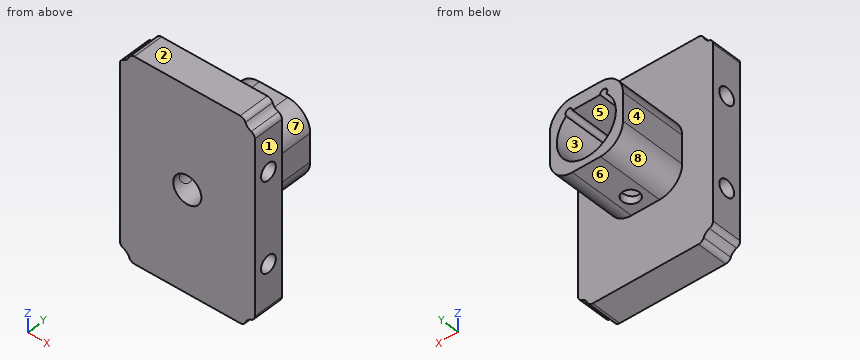
from build123d import *

# Parameters (mm, degrees)
EXTRUDE_1_DEPTH     = 12
EXTRUDE_3_DEPTH     = 5.5
SKETCH_6_R          = 1.5
CUT_EXTRUDE_2_DEPTH = 31
SKETCH_7_R          = 1.5
CUT_EXTRUDE_3_DEPTH = 31
SKETCH_8_R          = 2.5
CUT_EXTRUDE_5_DEPTH = 31
EXTRUDE_START       = -24
SKETCH_9_R          = 1.5
EXTRUDE_4_DEPTH     = 24
SKETCH_10_R         = 2.5
CUT_EXTRUDE_6_DEPTH = 24


with BuildPart() as part:
    # 草图1 → 凸台-拉伸1 (new body)
    with BuildSketch(Plane(origin=(0, 0, 0), x_dir=(1, 0, 0), z_dir=(0, 1, 0))):
        with BuildLine():
            ThreePointArc((6.5, -2.5), (5.328427125, -5.328427125), (2.5, -6.5))
            Line((2.5, -6.5), (-2.5, -6.5))
            ThreePointArc((-2.5, -6.5), (-5.328427125, -5.328427125), (-6.5, -2.5))
            Line((-6.5, -2.5), (-6.5, 2.5))
            ThreePointArc((-6.5, 2.5), (-5.328427125, 5.328427125), (-2.5, 6.5))
            Line((-2.5, 6.5), (2.5, 6.5))
            ThreePointArc((2.5, 6.5), (5.328427125, 5.328427125), (6.5, 2.5))
            Line((6.5, 2.5), (6.5, -2.5))
        make_face()
        with BuildLine():
            ThreePointArc((3.581278005, -3.838873253), (0, 5.25), (-3.581278005, -3.838873253))
            ThreePointArc((-3.581278005, -3.838873253), (-3.300605298, -4.858604348), (-2.435602742, -4.25))
            Line((-2.435602742, -4.25), (2.435602742, -4.25))
            ThreePointArc((2.435602742, -4.25), (3.300605298, -4.858604348), (3.581278005, -3.838873253))
        make_face(mode=Mode.SUBTRACT)
    extrude(amount=EXTRUDE_1_DEPTH)

    # 草图3 → 凸台-拉伸3 (add)
    with BuildSketch(Plane.XZ):
        with BuildLine():
            Line((12, 15.394651328), (12, -15.394651328))
            ThreePointArc((12, -15.394651328), (11.824116747, -15.961071302), (11.358336826, -16.328243701))
            ThreePointArc((11.358336826, -16.328243701), (10.733804764, -16.733804764), (10.328243701, -17.358336826))
            ThreePointArc((10.328243701, -17.358336826), (9.961071302, -17.824116747), (9.394651328, -18))
            Line((9.394651328, -18), (-9.394651328, -18))
            ThreePointArc((-9.394651328, -18), (-9.961071302, -17.824116747), (-10.328243701, -17.358336826))
            ThreePointArc((-10.328243701, -17.358336826), (-10.733804764, -16.733804764), (-11.358336826, -16.328243701))
            ThreePointArc((-11.358336826, -16.328243701), (-11.824116747, -15.961071302), (-12, -15.394651328))
            Line((-12, -15.394651328), (-12, 15.394651328))
            ThreePointArc((-12, 15.394651328), (-11.824116747, 15.961071302), (-11.358336826, 16.328243701))
            ThreePointArc((-11.358336826, 16.328243701), (-10.733804764, 16.733804764), (-10.328243701, 17.358336826))
            ThreePointArc((-10.328243701, 17.358336826), (-9.961071302, 17.824116747), (-9.394651328, 18))
            Line((-9.394651328, 18), (9.394651328, 18))
            ThreePointArc((9.394651328, 18), (9.961071302, 17.824116747), (10.328243701, 17.358336826))
            ThreePointArc((10.328243701, 17.358336826), (10.733804764, 16.733804764), (11.358336826, 16.328243701))
            ThreePointArc((11.358336826, 16.328243701), (11.824116747, 15.961071302), (12, 15.394651328))
        make_face()
    extrude(amount=EXTRUDE_3_DEPTH)

    # 草图6 → 切除-拉伸2 (cut)
    with BuildSketch(Plane.ZY.offset(12)):
        with Locations((0, -2.75)):
            Circle(SKETCH_6_R)
        with Locations((8, -2.75)):
            Circle(SKETCH_6_R)
        with Locations((-8, -2.75)):
            Circle(SKETCH_6_R)
    extrude(amount=-CUT_EXTRUDE_2_DEPTH, mode=Mode.SUBTRACT)

    # 草图7 → 切除-拉伸3 (cut)
    with BuildSketch(Plane.XY.offset(6.5)):
        with Locations((0, 3)):
            Circle(SKETCH_7_R)
    extrude(amount=-CUT_EXTRUDE_3_DEPTH, mode=Mode.SUBTRACT)

    # 草图8 → 切除-拉伸5 (cut)
    with BuildSketch(Plane.XZ.offset(5.5)):
        with Locations(Location((0, 0, 0), (0, 0, 270))):
            Circle(SKETCH_8_R)
    extrude(amount=-CUT_EXTRUDE_5_DEPTH, mode=Mode.SUBTRACT)

    # 草图9 → 凸台-拉伸4 (add)
    with BuildSketch(Plane(origin=(12, 0, 0), x_dir=(0, 0, -1), z_dir=(1, 0, 0)).offset(EXTRUDE_START)):
        with Locations(Location((0, -2.75, 0), (0, 0, 180))):
            Circle(SKETCH_9_R)
    extrude(amount=EXTRUDE_4_DEPTH)

    # 草图10 → 切除-拉伸6 (cut)
    with BuildSketch(Plane.XZ.offset(5.5)):
        with Locations(Location((0, 0, 0), (0, 0, 270))):
            Circle(SKETCH_10_R)
    extrude(amount=-CUT_EXTRUDE_6_DEPTH, mode=Mode.SUBTRACT)


solid = part.part
Design review of the part built by this model. Coordinates are the model's own, in mm. Face numbers are marked on the shaded views. A direction names the side the tool comes from. Give positions to 0.01 mm unless a question says otherwise; leave off trailing zeros. Order: outer loops, then holes, each group sorted by start corner. A loop starts at its lowest first (then second) coordinate and runs counter-clockwise, first axis right, second up. Notation, with made-up numbers: (-10, -19) - (10, -19) arc R18 ccw to (10, -8) - close; hole circle Ø5 at (-11, 27). An arc over 180 degrees is marked (long way). Use CSV: the item, a comma, the result in double quotes. Start each with the question number.
Q1. Take a section at C-C (y = -2.75). State the section outline as (x, z) points.
Q2. Take a section at D-D (z = 0). State the section outline as (x, y) points.
Q3. Draft analysis for pull direction X (two halves, no side actions). For the marked faces 1, 2 and 3, state which applies: pulls with the +X half, pulls with the -X half, needs draft (parallel to the pull), parting line crosses it, or undercut.
Q4. For line 1 (Y direction, x = 3.5, z = 8); line 2 (Z direction, x = 0, y = 6.25); line 3 (Z direction, x = -7, y = -3.75), list the stretches that pass through material, from the lowest coordinate up.
Q5. Machinability: for the marked faces 4, 5, 6, 7 and 8, which of the approach directions +Z, -Z, +X, -X, +Y, -Y give a long, thin tool a straight path to every point of the face, cutting with its end or side? Answer none if there is none.
Q6. Take a section at A-A (x = 0). State the section outline as (y, z) points.
Q7. Take a section at B-B (z = 8). State the section outline as (x, y) points, and give its area (3 significant figures).
Q8. For P1, Ø3, axis at x = 0, z = -10, coming from the +Y side; P2, Ø1.5, axis at y = 8.5, z = -1, coming from the -X side; P3, Ø1.5, axis at x = -3.08, z = 4.25, coming from the +Y side; P4, Ø4, axis at x = -0.5, y = 5.5, coming from the -Z side, all flat-tipped, find the tip position at first contact; note any pin that passes through.
Calculated:
1,outline,"(-12, -15.39) arc R1 ccw to (-11.36, -16.33) arc R1.79 cw to (-10.33, -17.36) arc R1 ccw to (-9.39, -18) - (9.39, -18) arc R1 ccw to (10.33, -17.36) arc R1.79 cw to (11.36, -16.33) arc R1 ccw to (12, -15.39) - (12, -9.5) - (-12, -9.5) - close; (-12, -6.5) - (12, -6.5) - (12, 6.5) - (-12, 6.5) - close; (-12, 9.5) - (12, 9.5) - (12, 15.39) arc R1 ccw to (11.36, 16.33) arc R1.79 cw to (10.33, 17.36) arc R1 ccw to (9.39, 18) - (-9.39, 18) arc R1 ccw to (-10.33, 17.36) arc R1.79 cw to (-11.36, 16.33) arc R1 ccw to (-12, 15.39) - close; hole circle Ø5 at (0, 0)"
2,outline,"(-12, -5.5) - (-2.5, -5.5) - (-2.5, 0) - (-5.25, 0) - (-5.25, 12) - (-6.5, 12) - (-6.5, 0) - (-12, 0) - close; (2.5, -5.5) - (12, -5.5) - (12, 0) - (6.5, 0) - (6.5, 12) - (5.25, 12) - (5.25, 0) - (2.5, 0) - close"
3,face 1,"pulls with the +X half"
3,face 2,"needs draft"
3,face 3,"undercut"
4,line 1,"y = -5.5 to -4.25, -1.25 to 0"
4,line 2,"z = -6.5 to -5.25, 4.25 to 6.5"
4,line 3,"z = -18 to -9.12, -6.88 to 6.88, 9.12 to 18"
5,face 4,"+Z, -Z, -X, +Y"
5,face 5,"+Y"
5,face 6,"-Z, +X, -X, +Y"
5,face 7,"+Z, +X, +Y"
5,face 8,"-Z, -X, +Y"
6,outline,"(-5.5, -18) - (0, -18) - (0, -6.5) - (1.5, -6.5) - (1.5, -5.25) - (0, -5.25) - (0, -2.5) - (-5.5, -2.5) - close; (-5.5, 2.5) - (0, 2.5) - (0, 4.25) - (1.5, 4.25) - (1.5, 6.5) - (0, 6.5) - (0, 18) - (-5.5, 18) - close; (4.5, -6.5) - (12, -6.5) - (12, -5.25) - (4.5, -5.25) - close; (4.5, 4.25) - (12, 4.25) - (12, 6.5) - (4.5, 6.5) - close; hole circle Ø3 at (-2.75, -8); hole circle Ø3 at (-2.75, 8)"
7,outline,"(-12, -5.5) - (12, -5.5) - (12, -4.25) - (-12, -4.25) - close; (-12, -1.25) - (12, -1.25) - (12, 0) - (-12, 0) - close"
7,area,"60.0 mm²"
8,P1,"stops at y = 0"
8,P2,"stops at x = -6.5"
8,P3,"stops at y = 12"
8,P4,"stops at z = -6.5"
